```python
from build123d import *

# Parameters (mm, degrees)
F1_DEPTH = 3.175


with BuildPart() as f1:
    # F0 (on Top) → F1 (new body)
    with BuildSketch(Plane.XY):
        Polygon((-12.7, 6.35), (-12.7, -101.6), (12.7, -101.6), (12.7, 4.7625), (3.175, 4.7625), (3.175, 14.2875), (12.7, 14.2875), (12.7, 101.6), (3.175, 101.6), (3.175, 95.25), (-3.175, 95.25), (-3.175, 101.6), (-12.7, 101.6), (-12.7, 15.875), (-3.175, 15.875), (-3.175, 6.35), align=None)
    extrude(amount=F1_DEPTH)


solid = f1.part
```
Input: part model. Units: mm. Frame: model coordinates. A direction names the side the tool comes from. Give positions to 0.01 mm unless a question says otherwise; leave off trailing zeros. Order: outer loops, then holes, each group sorted by start corner. A loop starts at its lowest first (then second) coordinate and runs counter-clockwise, first axis right, second up.
1. Set-up query: faces 5 (the face through (0, 95.25, 2)), 6 (the face through (8, 101.6, 2)), 7 (the face through (8, 14.288, 2)), 8 (the face through (-3.175, 11, 2)). Return all of +Z, -Z, +X, -X, +Y, -Y with unobstructed straight access to the full face (end or side cutting, diameter ignored); none if empty.
Computed:
face 5: +Z, -Z, +Y
face 6: +Z, -Z, +X, -X, +Y
face 7: +Z, -Z, +X
face 8: +Z, -Z, -X
2. Pin query (flat end, axial travel): pin 1 Ø1.6 at (x, z) = (1, 1.5) entering from +Y. Return the tip coordinate at first contact, or that it passes through.
Computed:
pin 1: stops at y = 95.25
3. Cut plane A-A (x = -6.75). Return loops of the section in (y, z) (3 decimals), and give its area (3 significant figures).
Computed:
outline: (-101.6, 0) - (6.35, 0) - (6.35, 3.175) - (-101.6, 3.175) - close; (15.875, 0) - (101.6, 0) - (101.6, 3.175) - (15.875, 3.175) - close
area: 615 mm2
4. Line query: probe 1 along Y at (x, z) = (-10.5, 1.4) (3 decimals); probe 2 along Y at (x, z) = (8.75, 1.1); probe 3 along X at (y, z) = (7.5, 0.8) (3 decimals). Output: solid intervals per line, ascending.
Computed:
probe 1: y = -101.6 to 6.35, 15.875 to 101.6
probe 2: y = -101.6 to 4.76, 14.29 to 101.6
probe 3: x = -3.175 to 3.175
5. Draft query along X for faces 1 (the face through (-3.175, 98, 2)), 2 (the face through (3.175, 9, 2)), 3 (the face through (3.175, 98, 2)), 4 (the face through (0, -101.6, 2)). Return one class per face: released by +X, released by -X, zero draft, split by the parting line, or undercut.
Computed:
face 1: undercut
face 2: released by +X
face 3: undercut
face 4: zero draft
